```python
from build123d import *

# Parameters (mm, degrees)
SKETCH_2_R               = 66.5
SKETCH_2_R_2             = 65.5
EXTRUDE_1_DEPTH          = 175
SKETCH_3_R               = 65.5
EXTRUDE_2_DEPTH          = 3
CUT_EXTRUDE_1_DEPTH      = 199.669323248
CUT_EXTRUDE_1_DEPTH_BACK = 199.669323248
SKETCH_4_W               = 50
SKETCH_4_H               = 77


with BuildPart() as part:
    # 스케치2 → 보스-돌출1 (new body)
    with BuildSketch(Plane(origin=(0, 0, 0), x_dir=(1, 0, 0), z_dir=(0, 1, 0))):
        with Locations(Location((0, 0, 0), (0, 0, 270))):
            Circle(SKETCH_2_R)
        with Locations(Location((0, 0, 0), (0, 0, 270))):
            Circle(SKETCH_2_R_2, mode=Mode.SUBTRACT)
    extrude(amount=EXTRUDE_1_DEPTH)

    # 스케치3 → 보스-돌출2 (add)
    with BuildSketch(Plane(origin=(0, 0, 0), x_dir=(1, 0, 0), z_dir=(0, 1, 0))):
        with Locations(Location((0, 0, 0), (0, 0, 270))):
            Circle(SKETCH_3_R)
    extrude(amount=EXTRUDE_2_DEPTH)

    # 스케치4 → 컷-돌출1 (cut, two sides: drawn at the far end of the back side and taken through both)
    with BuildSketch(Plane.XY.offset(-CUT_EXTRUDE_1_DEPTH_BACK)):
        with Locations((41.5, 49.5)):
            Rectangle(SKETCH_4_W, SKETCH_4_H)
    extrude(amount=CUT_EXTRUDE_1_DEPTH + CUT_EXTRUDE_1_DEPTH_BACK, mode=Mode.SUBTRACT)


solid = part.part
```
Could you check a few things on this model? Use its own coordinates, in mm. A direction names the side the tool comes from. Round coordinates to 2 decimals unless told otherwise and drop trailing zeros. Loops run counter-clockwise (first coordinate to the right, second up) from the corner with the lowest first, then second, coordinate; pieces in that order, holes last. Notation, with made-up numbers: (-22, -35.5) -> (-11, -35.5) arc R17 cw to (-11, -14.5) -> close; hole circle Ø4 at (-31.5, -22.5). An arc over 180 degrees is marked (long way). Put each result on its own line as item: value.
Q1. Which directions (+Z, -Z, +X, -X, +Y, -Y) give clear straight access to the entire face, cutting with the end or side of a thin tool? Please do faces 1 (the flat face through (65.5, 88, -5.1)), 2 (the flat face through (-49, 175, 44)).
Checks:
face 1: +Z, -Z, +X
face 2: +Z, -Z, +X, -X, +Y
Q2. I want a section at C-C on x = 48.5. Write out the boundary of the cut face in (y, z).
Checks:
outline: (0, -45.5) -> (11, -45.5) -> (11, -44.02) -> (3, -44.02) -> (3, 44.02) -> (11, 44.02) -> (11, 45.5) -> (0, 45.5) -> close; (88, -45.5) -> (175, -45.5) -> (175, -44.02) -> (88, -44.02) -> close; (88, 44.02) -> (175, 44.02) -> (175, 45.5) -> (88, 45.5) -> close
Q3. For pin 1 Ø6 at (x, y) = (-18.5, 112) entering from -Z; pin 2 Ø4 at (x, y) = (-52.5, 107) entering from -Z; pin 3 Ø8 at (y, z) = (121.5, -3.5) entering from -X, each with a flat end and sliding along its axis, tell me the tip position at first contact or that it passes through.
Checks:
pin 1: z = -64.67
pin 2: z = -43.27
pin 3: x = -66.5
Q4. I want a section at A-A on z = 0. Write out the boundary of the cut face in (x, y).
Checks:
outline: (-66.5, 0) -> (66.5, 0) -> (66.5, 11) -> (65.5, 11) -> (65.5, 3) -> (-65.5, 3) -> (-65.5, 175) -> (-66.5, 175) -> close; (65.5, 88) -> (66.5, 88) -> (66.5, 175) -> (65.5, 175) -> close
Q5. Thinking about a two-plate mould opening in X: for faces 3 (the cylindrical face through (-64.919, 86.275, -14.416)), 4 (the cylindrical face through (-63.942, 106.907, -14.199)), 5 (the flat face through (1, 0, -1)), which applies, pulls with the +X half, pulls with the -X half, needs draft (parallel to the pull), parting line crosses it, or undercut?
Checks:
face 3: parting line crosses it
face 4: undercut
face 5: needs draft
Q6. I want a section at B-B on x = 0. Write out the boundary of the cut face in (y, z), and give its area (3 significant figures).
Checks:
outline: (0, -66.5) -> (175, -66.5) -> (175, -65.5) -> (3, -65.5) -> (3, 65.5) -> (175, 65.5) -> (175, 66.5) -> (0, 66.5) -> close
area: 743 mm2
Q7. I want a section at D-D on y = 120.5. Write out the boundary of the cut face in (x, z).
Checks:
outline: circle Ø133 at (0, 0); hole circle Ø131 at (0, 0)
Q8. Please list where these lines run through material, in increasing order: line 1 (Z direction, x = 2, y = 142); line 2 (X direction, y = 116, z = 0); line 3 (Y direction, x = -23.5, z = 30). Write a range as from..to.
Checks:
line 1: -66.47..-65.47, 65.47..66.47
line 2: -66.5..-65.5, 65.5..66.5
line 3: 0..3
